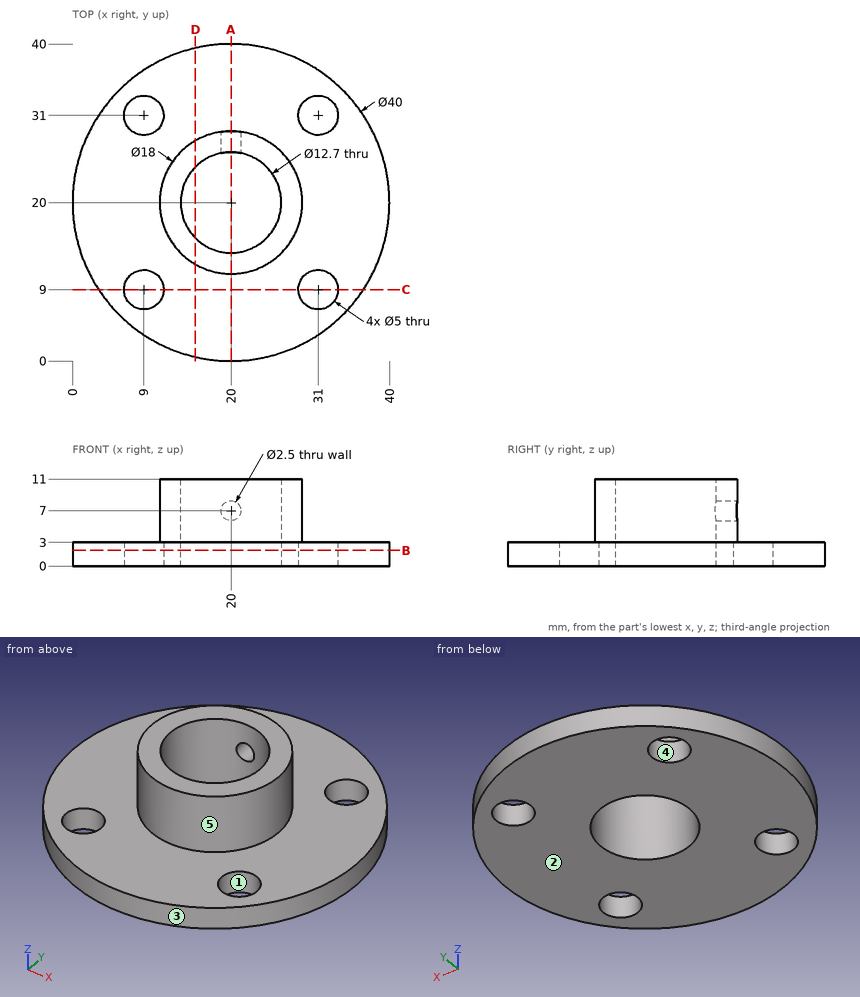
Answer from the drawing. Dimensions are ordinates in mm from the lowest x, y and z of the part. A direction names the side the tool comes from. Give positions to 0.01 mm unless a question says otherwise; leave off trailing zeros. Order: outer loops, then holes, each group sorted by start corner. A loop starts at its lowest first (then second) coordinate and runs counter-clockwise, first axis right, second up. Notation, with made-up numbers: (77, -35) -> (81, -35) arc R27 cw to (81, -7) -> close; hole circle Ø1 at (-40, -26.5). An arc over 180 degrees is marked (long way). One line per item, written item: value.
Item 1: Determine the mould class of the marked faces 1, 2 and 3 for opening direction X: released by +X, released by -X, zero draft, split by the parting line, or undercut.
Answer sheet:
face 1: undercut
face 2: zero draft
face 3: split by the parting line
Item 2: Find section A-A, the plane x = 20. Give the vertices of the cut face in (y, z).
Answer sheet:
outline: (0, 0) -> (13.65, 0) -> (13.65, 11) -> (11, 11) -> (11, 3) -> (0, 3) -> close; (26.35, 0) -> (40, 0) -> (40, 3) -> (29, 3) -> (29, 5.75) -> (26.35, 5.75) -> close; (26.35, 8.25) -> (29, 8.25) -> (29, 11) -> (26.35, 11) -> close
Item 3: Find section C-C, the plane y = 9. Give the vertices of the cut face in (x, z).
Answer sheet:
outline: (3.3, 0) -> (6.5, 0) -> (6.5, 3) -> (3.3, 3) -> close; (11.5, 0) -> (28.5, 0) -> (28.5, 3) -> (11.5, 3) -> close; (33.5, 0) -> (36.7, 0) -> (36.7, 3) -> (33.5, 3) -> close
Item 4: A tool of negligible diameter and unlimited length cuts with its end or side. For the marked faces 4 and 5, from which of +Z, -Z, +X, -X, +Y, -Y can it reach the whole face along a straight path? Write none if from no direction.
Answer sheet:
face 4: +Z, -Z
face 5: +Z
Item 5: Find section D-D, the plane x = 15.5. Give the vertices of the cut face in (y, z), plus the area to 3 significant figures.
Answer sheet:
outline: (0.51, 0) -> (15.52, 0) -> (15.52, 11) -> (12.21, 11) -> (12.21, 3) -> (0.51, 3) -> close; (24.48, 0) -> (39.49, 0) -> (39.49, 3) -> (27.79, 3) -> (27.79, 11) -> (24.48, 11) -> close
area: 143 mm²
Item 6: Straight lines are drawn through the part: probe 1 along Z at (x, y) = (37, 29.5); probe 2 along X at (y, z) = (19.5, 2.75); probe 3 along X at (y, z) = (15.5, 3.5). For each, find the intervals that lie inside material, in ascending order.
Answer sheet:
probe 1: 0 to 3
probe 2: 0.01 to 13.67, 26.33 to 39.99
probe 3: 12.21 to 15.52, 24.48 to 27.79
Item 7: Flat-ended cylindrical pins translate along their axes: P1, Ø4, axis at y = 34, z = 2, coming from the +X side; P2, Ø3, axis at x = 29, z = 3.5, coming from the -Y side; P3, Ø3, axis at x = 31, y = 31, coming from the +Z side; P4, Ø1.5, axis at x = 16, y = 30.5, coming from the +Z side. Find the tip coordinate at first contact, or state that the pin passes through.
Answer sheet:
P1: x = 36
P2: y = 1.49
P3: through
P4: z = 3
Item 8: Find section B-B, the plane z = 2. Give the vertices of the cut face in (x, y).
Answer sheet:
outline: circle Ø40 at (20, 20); hole circle Ø5 at (9, 9); hole circle Ø5 at (9, 31); hole circle Ø12.7 at (20, 20); hole circle Ø5 at (31, 9); hole circle Ø5 at (31, 31)
